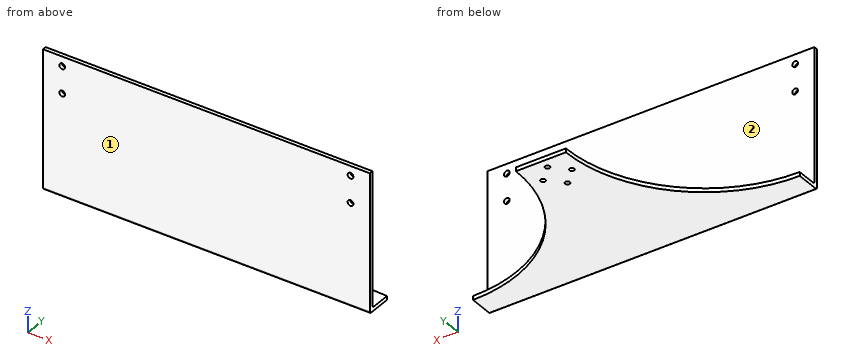
```python
from build123d import *

# Parameters (mm, degrees)
SKETCH1_W               = 170
SKETCH1_H               = 70
BOSS_EXTRUDE1_DEPTH     = 2
SKETCH2_R               = 1.5
CUT_EXTRUDE1_DEPTH      = 22
CUT_EXTRUDE1_DEPTH_BACK = 22
SKETCH4_W               = 170
SKETCH4_H               = 85
BOSS_EXTRUDE2_DEPTH     = 2
FILLET2_R               = 1
FILLET3_R               = 1
SKETCH6_R               = 1.25
CUT_EXTRUDE3_DEPTH      = 12
CUT_EXTRUDE3_DEPTH_BACK = 12
SKETCH5_R               = 72
CUT_EXTRUDE4_DEPTH      = 12
CUT_EXTRUDE4_DEPTH_BACK = 12


with BuildPart() as part:
    # Sketch1 → Boss-Extrude1 (new body)
    with BuildSketch(Plane(origin=(0, 0, 0), x_dir=(1, 0, 0), z_dir=(0, 1, 0))):
        with Locations((-0.557701395, -36.216789823)):
            Rectangle(SKETCH1_W, SKETCH1_H)
    extrude(amount=BOSS_EXTRUDE1_DEPTH)

    # Sketch2 → Cut-Extrude1 (cut, two sides)
    with BuildSketch(Plane(origin=(0, 2, 0), x_dir=(1, 0, 0), z_dir=(0, 1, 0))) as cut_extrude1_sk:
        with Locations((-75.557701395, -52.216789823)):
            Circle(SKETCH2_R)
        with Locations((-75.557701395, -66.216789823)):
            Circle(SKETCH2_R)
        with Locations((74.442298605, -52.216789823)):
            Circle(SKETCH2_R)
        with Locations((74.442298605, -66.216789823)):
            Circle(SKETCH2_R)
    extrude(amount=CUT_EXTRUDE1_DEPTH, mode=Mode.SUBTRACT)
    extrude(cut_extrude1_sk.sketch, amount=-CUT_EXTRUDE1_DEPTH_BACK, mode=Mode.SUBTRACT)

    # Sketch4 → Boss-Extrude2 (add)
    with BuildSketch(Plane(origin=(0, 0, 1.216789823), x_dir=(-1, 0, 0), z_dir=(0, 0, -1))):
        with Locations((0.557701395, 42.5)):
            Rectangle(SKETCH4_W, SKETCH4_H)
    extrude(amount=BOSS_EXTRUDE2_DEPTH)

    # Fillet2
    fillet2_edges = [part.edges().sort_by_distance(p)[0] for p in [
        (-0.557701395, 0, -0.783210177),
    ]]
    fillet(fillet2_edges, radius=FILLET2_R)

    # Fillet3
    fillet3_edges = [part.edges().sort_by_distance(p)[0] for p in [
        (-0.557701395, 2, 1.216789823),
    ]]
    fillet(fillet3_edges, radius=FILLET3_R)

    # Sketch6 → Cut-Extrude3 (cut, two sides)
    with BuildSketch(Plane.XY.offset(1.216789823)) as cut_extrude3_sk:
        with Locations((-0.557701395, 80)):
            Circle(SKETCH6_R)
        with Locations((-0.557701395, 65)):
            Circle(SKETCH6_R)
        with Locations((6.942298605, 72.5)):
            Circle(SKETCH6_R)
        with Locations((-8.057701395, 72.5)):
            Circle(SKETCH6_R)
    extrude(amount=CUT_EXTRUDE3_DEPTH, mode=Mode.SUBTRACT)
    extrude(cut_extrude3_sk.sketch, amount=-CUT_EXTRUDE3_DEPTH_BACK, mode=Mode.SUBTRACT)

    # Sketch5 → Cut-Extrude4 (cut, two sides)
    with BuildSketch(Plane.XY.offset(1.216789823)) as cut_extrude4_sk:
        with Locations((-85.557701395, 85)):
            Circle(SKETCH5_R)
        with Locations((84.442298605, 85)):
            Circle(SKETCH5_R)
    extrude(amount=CUT_EXTRUDE4_DEPTH, mode=Mode.SUBTRACT)
    extrude(cut_extrude4_sk.sketch, amount=-CUT_EXTRUDE4_DEPTH_BACK, mode=Mode.SUBTRACT)


solid = part.part
```
The model under review builds one solid part; all positions refer to its coordinate system, in mm. Face numbers are marked on the shaded views. A direction names the side the tool comes from. Round coordinates to 2 decimals unless told otherwise and drop trailing zeros. Loops run counter-clockwise (first coordinate to the right, second up) from the corner with the lowest first, then second, coordinate; pieces in that order, holes last. Notation, with made-up numbers: (42.5, 61) -> (70.5, 61) arc R30 cw to (70.5, 94) -> close; hole circle Ø7 at (48.25, -20). An arc over 180 degrees is marked (long way). Answer in a Markdown table with one row per item.
1) For pin 1 Ø3 at (x, y) = (-0.56, 80) entering from +Z; pin 2 Ø4 at (x, z) = (10.5, 29.5) entering from +Y, all flat-tipped, find the tip position at first contact; note any pin that passes through.
Taken from the geometry:
| item | result |
|---|---|
| pin 1 | stops at z = 1.22 |
| pin 2 | stops at y = 2 |
2) Consider section C-C, the plane z = 40. Write out the cut boundary in (x, y).
Taken from the geometry:
| item | result |
|---|---|
| outline | (-85.56, 0) -> (84.44, 0) -> (84.44, 2) -> (-85.56, 2) -> close |
3) Consider section A-A, the plane x = -4. Write out the cut boundary in (y, z), plus the area to 3 significant figures.
Taken from the geometry:
| item | result |
|---|---|
| outline | (0, 0.22) arc R1 ccw to (1, -0.78) -> (85, -0.78) -> (85, 1.22) -> (3, 1.22) arc R1 cw to (2, 2.22) -> (2, 71.22) -> (0, 71.22) -> close |
| area | 310 mm² |
4) Consider section B-B, the plane y = 48.5. Write out the cut boundary in (x, z).
Taken from the geometry:
| item | result |
|---|---|
| outline | (-23.5, -0.78) -> (22.38, -0.78) -> (22.38, 1.22) -> (-23.5, 1.22) -> close |
5) Wall thickness on line 1 along Y through (x, z) = (-51, 40); line 2 along Z through (x, y) = (-3, 64): over which ranges is each line inside the solid? List them lowest first.
Taken from the geometry:
| item | result |
|---|---|
| line 1 | y = 0 to 2 |
| line 2 | z = -0.78 to 1.22 |
6) Tool access review of the marked faces 1 and 2: name each direction out of +Z, -Z, +X, -X, +Y, -Y from which nothing blocks a thin tool from reaching the whole face with its end or side.
Taken from the geometry:
| item | result |
|---|---|
| face 1 | +Z, -Z, +X, -X, -Y |
| face 2 | +Z, +X, -X, +Y |
7) Consider section D-D, the plane x = 63. Write out the cut boundary in (y, z), plus the area to 3 significant figures.
Taken from the geometry:
| item | result |
|---|---|
| outline | (0, 0.22) arc R1 ccw to (1, -0.78) -> (16.27, -0.78) -> (16.27, 1.22) -> (3, 1.22) arc R1 cw to (2, 2.22) -> (2, 71.22) -> (0, 71.22) -> close |
| area | 173 mm² |
